Answer from the drawing. Dimensions are ordinates in mm from the lowest x, y and z of the part. Give positions to 0.01 mm unless a question says otherwise; leave off trailing zeros. Loops run counter-clockwise (first coordinate to the right, second up) from the corner with the lowest first, then second, coordinate; pieces in that order, holes last. Notation, with made-up numbers: M 88.5,38 L 147.5,38 A19 ccw 147.5,51 Z; hole C -32,-3.5 d6. An arc over 180 degrees is marked long. Return JSON: item names as keys, results as strings. Group by question number.
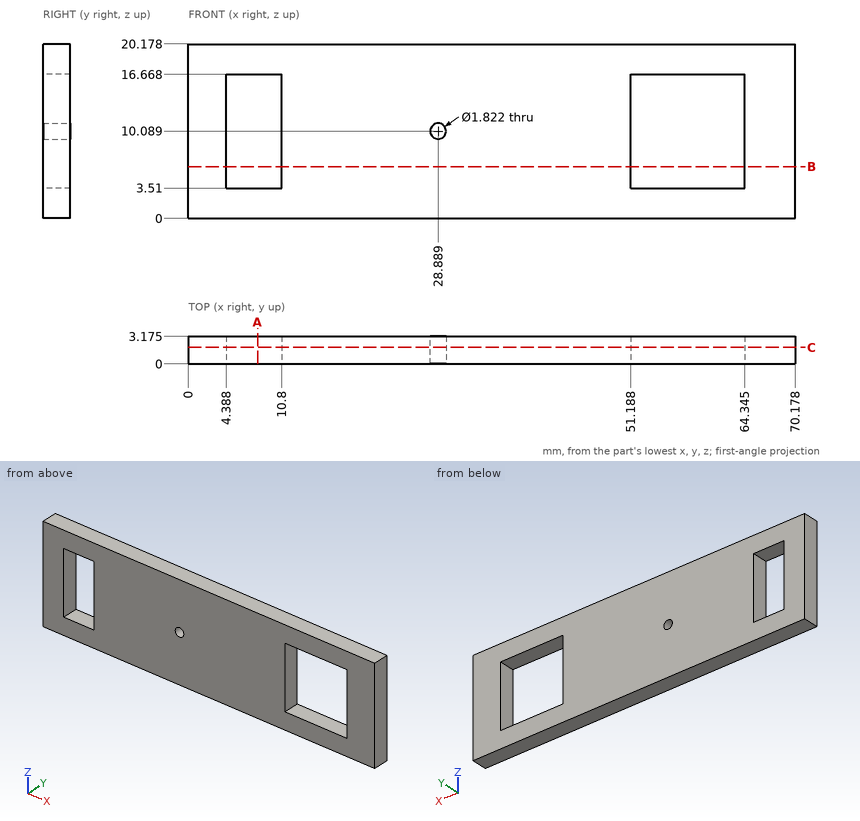
1. Straight lines are drawn through the part: line 1 along X through (y, z) = (2.35, 15) (1 decimal); line 2 along Z through (x, y) = (53, 1.55). For each, find the intervals that lie inside material, in ascending order.
2. Find section A-A (x = 8). Write down the section's boundary in (y, z) (1 decimal).
3. Find section B-B (z = 6). Write down the section's boundary in (x, y) (1 decimal), and give its area (3 significant figures).
4. Find section C-C (y = 1.9). Write down the section's boundary in (x, z) (1 decimal).
Result:
{
 "1": {"line 1": "x = 0 to 4.4, 10.8 to 51.2, 64.3 to 70.2", "line 2": "z = 0 to 3.51, 16.67 to 20.18"},
 "2": {"outline": "M 0,0 L 3.2,0 L 3.2,3.5 L 0,3.5 Z; M 0,16.7 L 3.2,16.7 L 3.2,20.2 L 0,20.2 Z"},
 "3": {"outline": "M 0,0 L 4.4,0 L 4.4,3.2 L 0,3.2 Z; M 10.8,0 L 51.2,0 L 51.2,3.2 L 10.8,3.2 Z; M 64.3,0 L 70.2,0 L 70.2,3.2 L 64.3,3.2 Z", "area": "161 mm2"},
 "4": {"outline": "M 0,0 L 70.2,0 L 70.2,20.2 L 0,20.2 Z; hole M 4.4,3.5 L 10.8,3.5 L 10.8,16.7 L 4.4,16.7 Z; hole C 28.9,10.1 d1.8; hole M 51.2,3.5 L 64.3,3.5 L 64.3,16.7 L 51.2,16.7 Z"}
}
